Can you work these out from the model? Positions are in its coordinate system, mm. Round coordinates to 2 decimals unless told otherwise and drop trailing zeros. Write each loop counter-clockwise with the first axis right and the second up, starting at its lowest first coordinate (ties: lowest second). Pieces come first, ordered by that corner, then holes. Notation, with made-up numbers: M -2,60 L 23,60 A19 cw 23,87 Z; hole C 21.5,-18.5 d7. An arc over 180 degrees is marked long. Answer in a Markdown table with one row per item. Add a question column.
(1) If I drill on probe 1 along X at (y, z) = (4.75, 20); probe 2 along X at (y, z) = (4.5, 27); probe 3 along Z at (x, y) = (-35, 3.5), over which ranges is the centre line in solid material (lowest first)?
(2) If we mould it in two halves opening along X, with no side actions, what happens to faces 1 (the face through (-1, 9.525, -1)), 2 (the face through (0.33, 4.7, -29.48)), 3 (the face through (45, 5, 1))? For each: released by +X, released by -X, zero draft, split by the parting line, or undercut.
(3) Suppose I cut it at C-C, the plane y = 8.25. Count the separate pieces of the cut face and the enclosed holes in it, then the cut area to 3 significant figures.
(4) Suppose I cut it at B-B, the plane x = 0. Write out the boundary of the cut face in (y, z) (3 decimals), then the cut area to 3 significant figures.
(5) Suppose I cut it at A-A, the plane z = -27. Write out the boundary of the cut face in (x, y) (3 decimals).
from build123d import *

# Parameters (mm, degrees)
SKETCH1_W                   = 90
SKETCH1_H                   = 75
BOSS_EXTRUDE1_DEPTH         = 9.525
M8_CLEARANCE_HOLE1_D        = 9
FIXED_M6X1_0_TAPPED_HOLE1_D = 5
M3X0_5_TAPPED_HOLE1_D       = 2.5
CHAMFER1_SIZE               = 1


with BuildPart() as part:
    # Sketch1 → Boss-Extrude1 (new body)
    with BuildSketch(Plane(origin=(0, 0, 0), x_dir=(1, 0, 0), z_dir=(0, 1, 0))):
        Rectangle(SKETCH1_W, SKETCH1_H)
    extrude(amount=BOSS_EXTRUDE1_DEPTH)

    # M8 Clearance Hole1 (through all)
    with Locations(Plane(origin=(0, 9.525, 0), x_dir=(1, 0, 0), z_dir=(0, 1, 0))):
        with Locations((-35, 20), (35, 20), (35, -20), (-35, -20)):
            Hole(M8_CLEARANCE_HOLE1_D / 2)

    # Fixed M6x1.0 Tapped Hole1 (through all)
    with Locations(Plane(origin=(0, 9.525, 0), x_dir=(1, 0, 0), z_dir=(0, 1, 0))):
        with Locations((-15, 27), (0, 27), (0, -27), (-15, -27)):
            Hole(FIXED_M6X1_0_TAPPED_HOLE1_D / 2)

    # M3x0.5 Tapped Hole1 (through all)
    with Locations(Plane(origin=(0, 9.525, 0), x_dir=(1, 0, 0), z_dir=(0, 1, 0))):
        with Locations((10.5, 33), (29.5, 33)):
            Hole(M3X0_5_TAPPED_HOLE1_D / 2)

    # Chamfer1
    chamfer1_edges = [part.edges().sort_by_distance(p)[0] for p in [
        (45, 4.7625, 37.5),
        (-45, 4.7625, 37.5),
        (-45, 4.7625, -37.5),
        (45, 4.7625, -37.5),
    ]]
    chamfer(chamfer1_edges, length=CHAMFER1_SIZE)


solid = part.part
Calculated:
| question | item | result |
|---|---|---|
| 1 | probe 1 | -45 to -39.5, -30.5 to 30.5, 39.5 to 45 |
| 1 | probe 2 | -45 to -17.5, -12.5 to -2.5, 2.5 to 45 |
| 1 | probe 3 | -37.5 to -24.5, -15.5 to 15.5, 24.5 to 37.5 |
| 2 | face 1 | zero draft |
| 2 | face 2 | undercut |
| 2 | face 3 | released by +X |
| 3 | separate pieces | 1 |
| 3 | enclosed holes | 10 |
| 3 | area | 6,410 mm² |
| 4 | outline | M 0,-37.5 L 9.525,-37.5 L 9.525,-29.5 L 0,-29.5 Z; M 0,-24.5 L 9.525,-24.5 L 9.525,24.5 L 0,24.5 Z; M 0,29.5 L 9.525,29.5 L 9.525,37.5 L 0,37.5 Z |
| 4 | area | 619 mm² |
| 5 | outline | M -45,0 L -17.5,0 L -17.5,9.525 L -45,9.525 Z; M -12.5,0 L -2.5,0 L -2.5,9.525 L -12.5,9.525 Z; M 2.5,0 L 45,0 L 45,9.525 L 2.5,9.525 Z |
